```python
from build123d import *

# Parameters (mm, degrees)
CROQUIS1_R              = 10
SALIENTE_EXTRUIR1_DEPTH = 71
CROQUIS2_R              = 5
CORTAR_EXTRUIR1_DEPTH   = 72
CROQUIS3_W              = 0.1
CROQUIS3_H              = 30


with BuildPart() as part:
    # Croquis1 → Saliente-Extruir1 (new body)
    with BuildSketch(Plane(origin=(0, 0, 0), x_dir=(1, 0, 0), z_dir=(0, 1, 0))):
        Circle(CROQUIS1_R)
    extrude(amount=SALIENTE_EXTRUIR1_DEPTH)

    # Croquis2 → Cortar-Extruir1 (cut, through all)
    with BuildSketch(Plane(origin=(0, 71, 0), x_dir=(1, 0, 0), z_dir=(0, 1, 0))):
        Circle(CROQUIS2_R)
    extrude(amount=-CORTAR_EXTRUIR1_DEPTH, mode=Mode.SUBTRACT)

    # Croquis3 → Cortar-Revolución1 (revolve, cut)
    with BuildSketch(Plane(origin=(0, 0, 0), x_dir=(0, 0, -1), z_dir=(1, 0, 0))):
        with Locations((9.95, 37.25)):
            Rectangle(CROQUIS3_W, CROQUIS3_H)
    revolve(axis=Axis((0, 71, 0), (0, -1, 0)), mode=Mode.SUBTRACT)


solid = part.part
```
Verification items for the finished model (mm, model axes). A direction names the side the tool comes from. Coordinates: 2 decimals unless noted, no trailing zeros. Loops run counter-clockwise (first coordinate to the right, second up) from the corner with the lowest first, then second, coordinate; pieces in that order, holes last. Notation, with made-up numbers: (-36.75, 34.5) -> (-9.75, 34.5) arc R16 ccw to (-9.75, 53.5) -> close; hole circle Ø8 at (35.5, 5.25). An arc over 180 degrees is marked (long way). Put each result on its own line as item: value.
1. Tool access check on faces 1 (the face through (-5, 0, 2)), 2 (the face through (2.974, 37.46, -9.443)). Record the directions out of +Z, -Z, +X, -X, +Y, -Y that give a thin tool (end or side, any length) a straight path to the whole face; none if there is none.
Result set:
face 1: +Z, -Z, +X, -X, -Y
face 2: none
2. Section check C-C, the plane z = -7. Record the boundary of the cut face in (x, y).
Result set:
outline: (-7.14, 0) -> (7.14, 0) -> (7.14, 22.25) -> (7, 22.25) -> (7, 52.25) -> (7.14, 52.25) -> (7.14, 71) -> (-7.14, 71) -> (-7.14, 52.25) -> (-7, 52.25) -> (-7, 22.25) -> (-7.14, 22.25) -> close
3. Section check A-A, the plane x = 0. Record the boundary of the cut face in (y, z).
Result set:
outline: (0, -10) -> (22.25, -10) -> (22.25, -9.9) -> (52.25, -9.9) -> (52.25, -10) -> (71, -10) -> (71, -5) -> (0, -5) -> close; (0, 5) -> (71, 5) -> (71, 10) -> (52.25, 10) -> (52.25, 9.9) -> (22.25, 9.9) -> (22.25, 10) -> (0, 10) -> close
4. Section check B-B, the plane y = 31. Record the boundary of the cut face in (x, z), then the cut area to 3 significant figures.
Result set:
outline: circle Ø19.8 at (0, 0); hole circle Ø10 at (0, 0)
area: 229 mm^2
5. Mould release check, pull along X, two halves, no side actions. Record for faces 3 (the face through (-1.08, 36, 4.88)), 4 (the face through (9.54, 10.97, -3)), 5 (the face through (-5, 71, 2)): pulls with the +X half, pulls with the -X half, needs draft (parallel to the pull), parting line crosses it, or undercut.
Result set:
face 3: undercut
face 4: parting line crosses it
face 5: needs draft
6. Gauge pin test, flat ends, axial feed: P1, Ø5, axis at x = -7.5, y = 55, coming from the +Z side; P2, Ø5, axis at x = 1, y = 29.5, coming from the +Z side; P3, Ø8, axis at x = 0, z = 0, coming from the -Y side; P4, Ø2, axis at x = -4.5, y = 33.5, coming from the -Z side. Record the tip position at first contact, or that the pin passes through.
Result set:
P1: stops at z = 8.66
P2: stops at z = 9.9
P3: passes through
P4: stops at z = -9.26
7. Section check D-D, the plane x = 7. Record the boundary of the cut face in (y, z).
Result set:
outline: (0, -7.14) -> (22.25, -7.14) -> (22.25, -7) -> (52.25, -7) -> (52.25, -7.14) -> (71, -7.14) -> (71, 7.14) -> (52.25, 7.14) -> (52.25, 7) -> (22.25, 7) -> (22.25, 7.14) -> (0, 7.14) -> close
8. Thickness scan on line 1 (X direction, y = 57.5, z = 0); line 2 (X direction, y = 24.5, z = 0). Record the ranges inside material, lowest first.
Result set:
line 1: x = -10 to -5, 5 to 10
line 2: x = -9.9 to -5, 5 to 9.9
